Autodesk Inventor part; units mm, degrees
ref_plane "YZ Plane" through (0, 0, 0) normal (1, 0, 0) x (0, 1, 0)
ref_plane "XZ Plane" through (0, 0, 0) normal (0, 1, 0) x (-1, 0, 0)
ref_plane "XY Plane" through (0, 0, 0) normal (0, 0, 1) x (1, 0, 0)
sketch "Sketch1" plane through (0, 0, 0) normal (0, 1, 0) x (-1, 0, 0)
  circle A0 centre (0.2636, -10.4031) radius 3.175
  line L0 (0.2636, -10.4031) -> (6.9811, -3.6856)
  line L1 (0.2636, -10.4031) -> (6.0619, -16.2014)
  line L2 (0.2636, -10.4031) -> (-5.5347, -4.6048)
  line L3 (0.2636, -10.4031) -> (-6.4539, -17.1206)
  circle A1 centre (6.9811, -3.6856) radius 1.75
  circle A2 centre (6.0619, -16.2014) radius 1.75
  circle A3 centre (-6.4539, -17.1206) radius 1.75
  circle A4 centre (-5.5347, -4.6048) radius 1.75
  circle A5 centre (0.2636, -10.4031) radius 14.1446
  circle A6 centre (6.9811, -3.6856) radius 4.445
  circle A7 centre (-6.4539, -17.1206) radius 4.445
  line L4 (3.838, -0.5425) -> (-9.597, -13.9775)
  line L5 (10.1242, -6.8287) -> (-3.3108, -20.2637)
  circle A8 centre (6.9811, -3.6856) radius 2.3813
  point P0 (0, 0)
  dimension "d3" = 9.5
  dimension "d4" = 90
  dimension "d5" = 90
  dimension "d6" = 90
  dimension "d7" = 3.5
  dimension "d8" = 3.5
  dimension "d9" = 3.5
  dimension "d10" = 3.5
  dimension "d12" = 8.89
  dimension "d13" = 8.89
  dimension "d18" = 4.7625
extrude "Extrusion2" add sketch "Sketch1" along normal blind 3.175 contours A0 L0 A6 L5 L1 | A0 L2 L4 A6 L0 | L1 L5 A7 L3 A0 | A0 L3 A7 L4 L2 | A8 | A6 | A7
sketch "Sketch3" plane through (0, 3.175, 0) normal (0, 1, 0) x (1, 0, 0)
  circle A0 centre (-6.9811, 3.6856) radius 1.75
  line L0 (-6.9811, 3.6856) -> (-6.9811, 13.6529)
  arc A1 (-11.4261, 3.6856) -> (-3.838, 0.5425) centre (-6.9811, 3.6856) ccw
  arc A2 (-10.126, 3.2493) -> (-4.7361, 1.4405) centre (-6.9811, 3.6856) ccw
  circle A3 centre (6.4539, 17.1206) radius 1.75
  arc A4 (8.699, 14.8755) -> (6.8902, 20.2655) centre (6.4539, 17.1206) ccw
  arc A5 (9.597, 13.9775) -> (6.4539, 21.5656) centre (6.4539, 17.1206) ccw
  line L1 (-3.838, 0.5425) -> (9.597, 13.9775)
  line L2 (-3.838, 0.5425) -> (9.597, 13.9775)
  line L3 (-4.7361, 1.4405) -> (8.699, 14.8755)
  arc A6 (-10.1242, 6.8287) -> (-3.838, 0.5425) centre (-6.9811, 3.6856) ccw
  line L4 (6.8902, 20.2655) -> (6.4539, 21.5656)
  line L5 (-10.126, 3.2493) -> (-11.4261, 3.6856)
  point P0 (0, 0)
extrude "Extrusion3" add sketch "Sketch3" along normal blind 25.4 contours L5 A2 L3 A4 L4 A5 L1 A1
sketch "Sketch4" plane through (0, 28.575, 0) normal (0, 1, 0) x (1, 0, 0)
  circle A0 centre (-6.9811, 3.6856) radius 1.75
  circle A1 centre (-6.9811, 3.6856) radius 4.445
  circle A2 centre (6.4539, 17.1206) radius 1.75
  circle A3 centre (6.4539, 17.1206) radius 4.445
  arc A4 (-11.4261, 3.6856) -> (-3.838, 0.5425) centre (-6.9811, 3.6856) ccw
  line L0 (-3.838, 0.5425) -> (9.597, 13.9775)
  line L1 (3.3108, 20.2637) -> (-10.1242, 6.8287)
  line L2 (-10.1242, 6.8287) -> (3.3108, 20.2637)
  point P0 (0, 0)
extrude "Extrusion4" add sketch "Sketch4" along normal blind 31.75 contours A0 | A1 | A1 L1 A3 L0 | A3 | A2
properties part number "Drone_leg"
Build history of the part. All positions in model axes, mm. A direction names the side the tool comes from. Round coordinates to 2 decimals unless told otherwise and drop trailing zeros. Order: outer loops, then holes, each group sorted by start corner. A loop starts at its lowest first (then second) coordinate and runs counter-clockwise, first axis right, second up. Notation, with made-up numbers: M 52,9 L 65,9 A15 ccw 65,26 Z; hole C 69.5,47 d3. An arc over 180 degrees is marked long. Use CSV: the item, a comma, the result in double quotes. Start each with the question number.
(1) Mould opens along Y. For faces 5 (the face through (-3.313, 44.228, -13.64)), 6 (the face through (0, 60.325, -11)), 7 (the face through (9.448, 15.697, -18.177)) say: +Y half, -Y half, draft (parallel to the pull), parting line (faces both ways), or undercut.
(2) Tool access for faces 1 (the face through (0.15, 1.57, -13.55)), 2 (the face through (-7.94, 15.7, -0.66)), 3 (the face through (2.79, 29.74, -7.17)), 4 (the face through (6.675, 15.697, -20.906)): list every direction of +Z, -Z, +X, -X, +Y, -Y with a clear straight run to the whole face (end or side of a thin tool).
(3) Cut at B-B on x = -0.5. List the corners of the cut face in (y, z) (1 decimal).
(4) Cut at A-A on z = -11.25. List the corners of the cut face in (x, y) (1 decimal), then the cut area to 3 significant figures.
(5) Flat gauge pins, fed straight in: P1, Ø5, axis at x = 0, y = 7, coming from the -Z side; P2, Ø1, axis at x = 7.5, y = 12, coming from the -Z side; P3, Ø5, axis at y = 7.5, z = -8.5, coming from the -X side. Where does each tip first touch, or does it go through?
(6) Cut at D-D on x = -7. List the corners of the cut face in (y, z) (1 decimal).
(7) Cut at C-C on y = 11.5. List the corners of the cut face in (x, z) (1 decimal), then the cut area to 3 significant figures.
(8) Drill centre lines: probe 1 along Y at (x, z) = (2.75, -16) (3 decimals); probe 2 along Z at (x, y) = (8.75, 26); probe 3 along Y at (x, z) = (6.5, -16.5) (3 decimals). Where is each one in solid material? Low to high.
Findings:
1,face 5,"draft"
1,face 6,"+Y half"
1,face 7,"undercut"
2,face 1,"-Y"
2,face 2,"-Z"
2,face 3,"+Z, +X, +Y, -Y"
2,face 4,"-X"
3,outline,"M 0,-16.5 L 3.2,-16.5 L 3.2,-13.6 L 0,-13.6 Z; M 0,-7.2 L 3.2,-7.2 L 3.2,-5.7 L 28.6,-5.7 L 28.6,-16.5 L 60.3,-16.5 L 60.3,-3.9 L 0,-3.9 Z"
4,outline,"M -5.7,0 L -3.3,0 L -3.3,3.2 L -5.7,3.2 Z; M -5.7,28.6 L 5.1,28.6 L 5.1,3.2 L 2.8,3.2 L 2.8,0 L 6.9,0 L 6.9,60.3 L -5.7,60.3 Z"
4,area,"465 mm^2"
5,P1,"stops at z = -8.68"
5,P2,"stops at z = -21.53"
5,P3,"stops at x = -0.18"
6,outline,"M 0,-10 L 3.2,-10 L 3.2,-5.4 L 0,-5.4 Z; M 0,-1.9 L 3.2,-1.9 L 3.2,-0.5 L 28.6,-0.5 L 28.6,-10 L 60.3,-10 L 60.3,0.8 L 0,0.8 Z"
7,outline,"M -11.4,-3.7 L -10.1,-3.2 A3.2 cw -4.7,-1.4 L 8.7,-14.9 A3.2 cw 6.9,-20.3 L 6.5,-21.6 A4.4 ccw 9.6,-14 L -3.8,-0.5 A4.4 ccw Z"
7,area,"46.4 mm^2"
8,probe 1,"y = 0 to 3.175, 28.575 to 60.325"
8,probe 2,"z = -20.93 to -19.31, -14.93 to -13.13"
8,probe 3,"y = 28.575 to 60.325"
